Model file for the job. Use its own axes, mm. Face numbers are marked on the shaded views. A direction names the side the tool comes from. Coordinates: 2 decimals unless noted, no trailing zeros. Loops run counter-clockwise (first coordinate to the right, second up) from the corner with the lowest first, then second, coordinate; pieces in that order, holes last. Notation, with made-up numbers: M 34,7 L 76,7 A30 cw 76,40 Z; hole C 75,62.5 d9. An arc over 180 degrees is marked long. Write item = value, one per line. Start each with the question number.
from build123d import *

# Parameters (mm, degrees)
SKETCH_1_R      = 4
EXTRUDE_2_DEPTH = 9
SKETCH_1_6_R    = 10
SKETCH_1_6_R_2  = 4
EXTRUDE_3_DEPTH = 3.5


with BuildPart() as part:
    # 草图1 → 凸台-拉伸2 (new, symmetric)
    with BuildSketch(Plane.XY):
        Circle(SKETCH_1_R)
    extrude(amount=EXTRUDE_2_DEPTH, both=True)

    # 草图1<6> → 凸台-拉伸3 (add, symmetric)
    with BuildSketch(Plane.XY):
        Circle(SKETCH_1_6_R)
        Circle(SKETCH_1_6_R_2, mode=Mode.SUBTRACT)
    extrude(amount=EXTRUDE_3_DEPTH, both=True)


solid = part.part
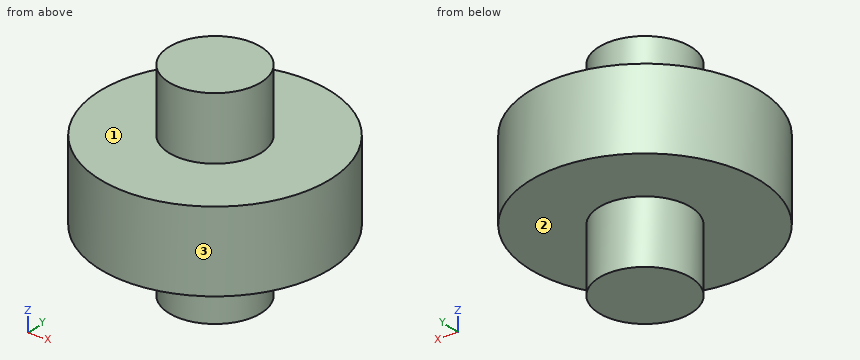
Item 1: Pin check, flat tips, straight feed: pin 1 Ø1 at (x, z) = (-3, 6.5) entering from +Y; pin 2 Ø1.5 at (x, y) = (3, 3.5) entering from -Z; pin 3 Ø8 at (y, z) = (4, -6) entering from -X; pin 4 Ø1 at (y, z) = (4, -1) entering from -X. Stop position of each tip, or through.
Item 2: Cut at C-C (z = -4.75). Give the cut face in (x, y).
Item 3: Cut at A-A (x = 0). Give the cut face in (y, z), plus the area to 3 significant figures.
Item 4: Cut at D-D (z = -0.5). Give the cut face in (x, y), plus the area to 3 significant figures.
Item 5: 3-axis set-ups, long thin cutter, end or side, ignore diameter. For the marked faces 1, 2 and 3: which of +Z, -Z, +X, -X, +Y, -Y reach the whole face in a straight line?
Item 6: Probe L1, parallel to Z at x = 4, y = -7.75; L2, parallel to X at y = 9, z = 2.75; L3, parallel to X at y = 2.75, z = 5.25. List the from-to ranges inside material, lowest first.
Reported:
q1.pin_1 = 3.12
q1.pin_2 = -9
q1.pin_3 = -9.96
q1.pin_4 = -9.37
q2.outline = C 0,0 d8
q3.outline = M -10,-3.5 L -4,-3.5 L -4,-9 L 4,-9 L 4,-3.5 L 10,-3.5 L 10,3.5 L 4,3.5 L 4,9 L -4,9 L -4,3.5 L -10,3.5 Z
q3.area = 228 mm^2
q4.outline = C 0,0 d20
q4.area = 314 mm^2
q5.face_1 = +Z
q5.face_2 = -Z
q5.face_3 = +Z, -Z
q6.L1 = -3.5 to 3.5
q6.L2 = -4.36 to 4.36
q6.L3 = -2.9 to 2.9
